Answer from the drawing. Dimensions are ordinates in mm from the lowest x, y and z of the part. Coordinates: 2 decimals unless noted, no trailing zeros. Loops run counter-clockwise (first coordinate to the right, second up) from the corner with the lowest first, then second, coordinate; pieces in that order, holes last. Notation, with made-up numbers: (-22, 54) - (-15, 54) arc R19 ccw to (-15, 59) - close; hole circle Ø2 at (-10.5, -26). An arc over 180 degrees is marked (long way). Write each question's results on one line, items separated by ' | '. Start each with the question number.
1. Find the intervals of material crossed by line 1 along Z through (x, y) = (22.5, 35.5); line 2 along Z through (x, y) = (23.25, 31); line 3 along Z through (x, y) = (13.75, 11), in increasing order. Write a range as [from, to].
2. Determine the mould class of the marked faces 1, 2 and 3 for opening direction X: released by +X, released by -X, zero draft, split by the parting line, or undercut.
3. A cutting plane is placed at B-B on x = 22.5. Determine the outline of the cut face in (y, z).
4. A cutting plane is placed at A-A on z = 3. Determine the outline of the cut face in (x, y).
5. A cutting plane is placed at D-D on x = 11. Determine the outline of the cut face in (y, z).
6. Each of these flat-tipped pins is pushed along its axis until it touches: P1, Ø1, axis at x = 17.5, y = 39.5, coming from the -Z side; P2, Ø3, axis at x = 22.5, z = 3, coming from the +Y side; P3, Ø10, axis at x = 6, y = 42, coming from the +Z side. Where does it stop, or does it pass through?
7. A cutting plane is placed at C-C on y = 5.5. Determine the outline of the cut face in (x, z).
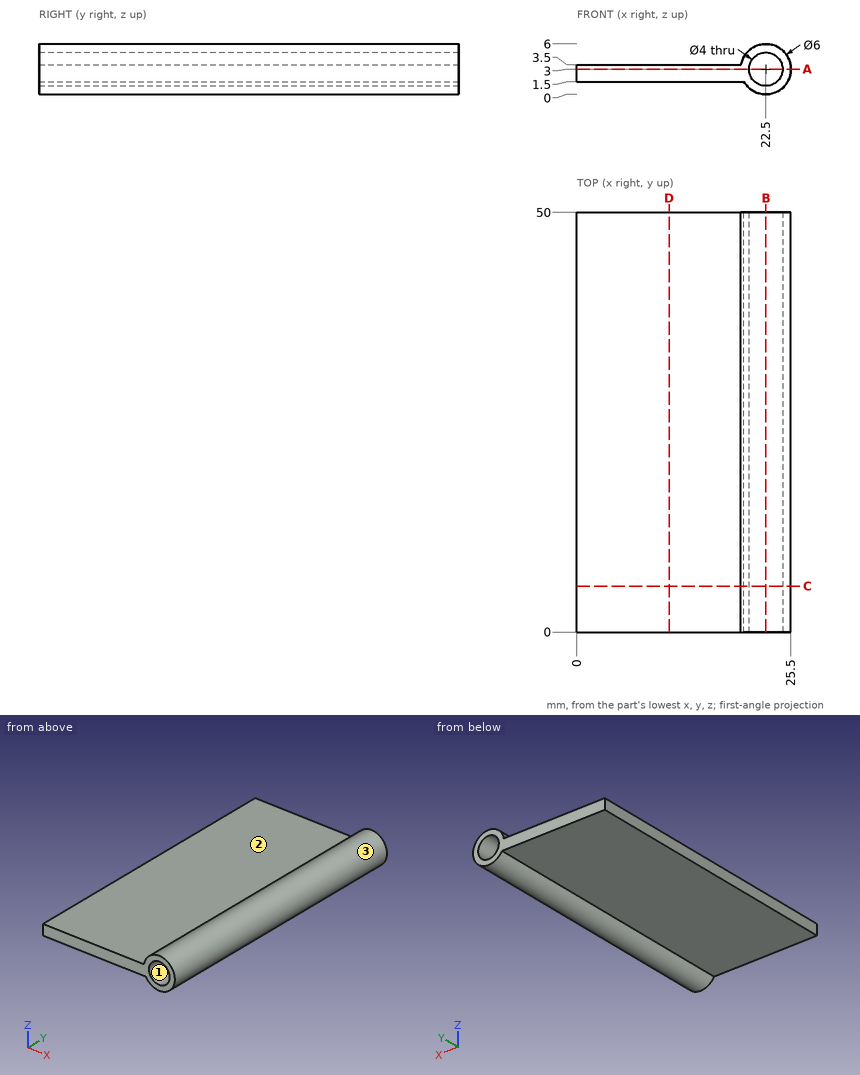
Values:
1) line 1: [0, 1], [5, 6] | line 2: [0.1, 1.15], [4.85, 5.9] | line 3: [1.5, 3.5]
2) face 1: undercut | face 2: zero draft | face 3: split by the parting line
3) outline: (0, 0) - (50, 0) - (50, 1) - (0, 1) - close; (0, 5) - (50, 5) - (50, 6) - (0, 6) - close
4) outline: (0, 0) - (20.5, 0) - (20.5, 50) - (0, 50) - close; (24.5, 0) - (25.5, 0) - (25.5, 50) - (24.5, 50) - close
5) outline: (0, 1.5) - (50, 1.5) - (50, 3.5) - (0, 3.5) - close
6) P1: z = 1.5 | P2: through | P3: z = 3.5
7) outline: (0, 1.5) - (19.9, 1.5) arc R3 ccw (long way) to (19.54, 3.5) - (0, 3.5) - close; hole circle Ø4 at (22.5, 3)
